Build history of the part. All positions in model axes, mm. A direction names the side the tool comes from. Round coordinates to 2 decimals unless told otherwise and drop trailing zeros. Order: outer loops, then holes, each group sorted by start corner. A loop starts at its lowest first (then second) coordinate and runs counter-clockwise, first axis right, second up. Notation, with made-up numbers: M 88,-12 L 113,-12 A14 ccw 113,5 Z; hole C 78,-23.5 d8. An arc over 180 degrees is marked long. One line per item, written item: value. Start each with the question number.
Item 1: Band-saw the part on D-D, the plane z = -10. Write the cut outline in (x, y), then the cut area to 3 significant figures.
Item 2: Tool access for faces 1 (the flat face through (-11.5, 0.1, 0)), 2 (the flat face through (0, -13.35, 37)), 3 (the flat face through (11.4, 0.1, 0)), 4 (the cylindrical face through (-4.086, 13.857, 18.564)): list every direction of +Z, -Z, +X, -X, +Y, -Y with a clear straight run to the whole face (end or side of a thin tool).
Item 3: Probe L1, parallel to Z at x = 0, y = 14; L2, parallel to Y at x = 13, z = 39; L3, parallel to X at y = 0.25, z = -7.5. List the from-to ranges inside material, lowest first.
Item 4: Two-plate mould, pull along Z, no slides. Class faces 5 (the cylindrical face through (-4.086, -13.843, 18.564)), 6 (the cylindrical face through (1.19, -0.01, 68.83)), 7 (the flat face through (0, 0.5, 59)): +Z half, -Z half, draft (parallel to the pull), parting line (faces both ways), or undercut.
Item 5: Band-saw the part on A-A, the plane z = 43. Write the cut outline in (x, y), then the cut area to 3 significant figures.
Item 6: Pin check, flat tips, straight feed: pin 1 (12 mm diameter, centred on x = -4.5, z = 31, fed in from +Y); pin 2 (5 mm diameter, centred on y = -5, z = -11, fed in from +X); pin 3 (1.5 mm diameter, centred on y = 6.5, z = 56, fed in from -X). Stop position of each tip, or through.
Item 7: Band-saw the part on B-B, the plane y = 1.5. Write the cut outline in (x, z).
Item 8: Band-saw the part on C-C, the plane x = 25. Write the cut outline in (y, z).
```python
from build123d import *

# Parameters (mm, degrees)
F1_R     = 18.85
F2_DEPTH = 13.35
F1_R_2   = 19.85
F3_DEPTH = 14.35
F4_DEPTH = 34.2
F5_DEPTH = 30
F6_DEPTH = 20.9
F1_R_3   = 31.8850678314
F8_DEPTH = 0.5


with BuildPart() as f2:
    # F1 (on Front) → F2 (new body, symmetric)
    with BuildSketch(Plane.XZ):
        with Locations((0, 36.9661189616)):
            Circle(F1_R)
    extrude(amount=F2_DEPTH, both=True)

    # F1 (on Front) → F3 (join, symmetric)
    with BuildSketch(Plane.XZ):
        with Locations((0, 36.9661189616)):
            Circle(F1_R_2)
        with Locations((0, 36.9661189616)):
            Circle(F1_R, mode=Mode.SUBTRACT)
    extrude(amount=F3_DEPTH, both=True)



with BuildPart() as f4:
    # F0 (on Top) → F4 (new body)
    with BuildSketch(Plane.XY):
        with BuildLine():
            ThreePointArc((5.4e-09, -11.15), (7.8842406121, -7.8842406083), (11.15, 0))
            ThreePointArc((11.15, 0), (7.8842406263, 7.8842405941), (4.56e-08, 11.15))
            ThreePointArc((4.56e-08, 11.15), (-11.15, 2.01e-08), (5.4e-09, -11.15))
        make_face()
        with BuildLine():
            ThreePointArc((4.56e-08, 11.15), (7.8842406263, 7.8842405941), (11.15, 0))
            ThreePointArc((11.15, 0), (7.8842406121, -7.8842406083), (5.4e-09, -11.15))
            Line((5.4e-09, -11.15), (9.0332718325, -11.15))
            ThreePointArc((9.0332718325, -11.15), (12.9527979757, -6.1763682372), (14.35, 0))
            ThreePointArc((14.35, 0), (12.9527979757, 6.1763682372), (9.0332718325, 11.15))
            Line((9.0332718325, 11.15), (4.56e-08, 11.15))
        make_face()
        with BuildLine():
            ThreePointArc((5.4e-09, -11.15), (-11.15, 2.01e-08), (4.56e-08, 11.15))
            Line((4.56e-08, 11.15), (-9.0332718325, 11.15))
            ThreePointArc((-9.0332718325, 11.15), (-12.9527979757, 6.1763682372), (-14.35, 0))
            ThreePointArc((-14.35, 0), (-12.9527979757, -6.1763682372), (-9.0332718325, -11.15))
            Line((-9.0332718325, -11.15), (5.4e-09, -11.15))
        make_face()
    extrude(amount=F4_DEPTH)

    # F0 (on Top) → F5 (join)
    with BuildSketch(Plane.XY):
        with BuildLine():
            ThreePointArc((5.4e-09, -11.15), (7.8842406121, -7.8842406083), (11.15, 0))
            ThreePointArc((11.15, 0), (7.8842406263, 7.8842405941), (4.56e-08, 11.15))
            ThreePointArc((4.56e-08, 11.15), (-11.15, 2.01e-08), (5.4e-09, -11.15))
        make_face()
    extrude(amount=-F5_DEPTH)


with BuildPart() as f6:
    # F1 (on Front) → F6 (new body, symmetric)
    with BuildSketch(Plane.XZ):
        with Locations((0, 36.9661189616)):
            Circle(F1_R_2)
        with Locations((0, 36.9661189616)):
            Circle(F1_R, mode=Mode.SUBTRACT)
        with Locations((0, 36.9661189616)):
            Circle(F1_R)
    extrude(amount=F6_DEPTH, both=True)


with BuildPart() as f4_1:
    add(f4.part)

    # F7: cut F6
    add(f6.part, mode=Mode.SUBTRACT)


with BuildPart() as f2_1:
    add(f2.part)

    add(f4_1.part)  # F8 merges F4
    # F1 (on Front) → F8 (join, symmetric)
    with BuildSketch(Plane.XZ):
        with Locations((0, 36.9661189616)):
            Circle(F1_R_3)
        with Locations((0, 36.9661189616)):
            Circle(F1_R_2, mode=Mode.SUBTRACT)
    extrude(amount=F8_DEPTH, both=True)


solid = f2_1.part
```
Output:
1. outline: C 0,0 d22.3
1. area: 391 mm²
2. face 1: -Z, -X
2. face 2: -Y
2. face 3: -Z, +X
2. face 4: +Y
3. L1: z = 17.12 to 18.12, 55.82 to 56.82
3. L2: y = -13.35 to 13.35
3. L3: x = -11.15 to 11.15
4. face 5: undercut
4. face 6: parting line
4. face 7: draft
5. outline: M -31.31,-0.5 L -18.91,-0.5 L -18.91,-14.35 L -17.86,-14.35 L -17.86,-13.35 L 17.86,-13.35 L 17.86,-14.35 L 18.91,-14.35 L 18.91,-0.5 L 31.31,-0.5 L 31.31,0.5 L 18.91,0.5 L 18.91,14.35 L 17.86,14.35 L 17.86,13.35 L -17.86,13.35 L -17.86,14.35 L -18.91,14.35 L -18.91,0.5 L -31.31,0.5 Z
5. area: 1,040 mm²
6. pin 1: stops at y = 13.35
6. pin 2: stops at x = 10.87
6. pin 3: stops at x = -7.73
7. outline: M -14.27,0 L -11.05,0 L -11.05,-30 L 11.05,-30 L 11.05,0 L 14.27,0 L 14.27,23.17 A19.85 ccw long -14.27,23.17 Z
8. outline: M -0.5,17.18 L 0.5,17.18 L 0.5,56.76 L -0.5,56.76 Z
